CAD build for the part. Positions are in the model's coordinates, mm. Face numbers are marked on the shaded views. Coordinates: 2 decimals unless noted, no trailing zeros. Loops run counter-clockwise (first coordinate to the right, second up) from the corner with the lowest first, then second, coordinate; pieces in that order, holes last. Notation, with made-up numbers: (25, -22) - (52, -22) arc R30 cw to (52, 8) - close; hole circle Ø1 at (49, -11.75). An arc over 180 degrees is marked (long way). Put each result on its own line as item: value.
```python
from build123d import *

# Parameters (mm, degrees)
F0_R     = 12
F1_DEPTH = 6
F2_R     = 18
F3_DEPTH = 2
F5_D     = 1.5
F6_R     = 4
F7_DEPTH = 8.001
F9_D     = 2.5
F9_DEPTH = 18.001


with BuildPart() as f1:
    # F0 (on Top) → F1 (new body)
    with BuildSketch(Plane.XY):
        Circle(F0_R)
    extrude(amount=F1_DEPTH)

    # F2 (on face) → F3 (join)
    with BuildSketch(Plane.XY.offset(6)):
        Circle(F2_R)
    extrude(amount=F3_DEPTH)

    # F5 (through all)
    with Locations(Plane.XY.offset(8)):
        with Locations((-17, 0), (-16.4659137392, 4.2277280818), (-14.8972135607, 8.1898124597), (-12.3924666662, 11.6373008008), (-9.1090555146, 14.3535747335), (-5.2532889044, 16.167960777), (-1.067438832, 16.9664543833), (3.185482348, 16.6988832624), (7.2382479566, 15.3820598919), (10.8362078257, 13.0987251272), (13.7532889044, 9.992349289), (15.8062002601, 6.2581173956), (-16.4659137392, -4.2277280818), (-14.8972135607, -8.1898124597), (-12.3924666662, -11.6373008008), (-9.1090555146, -14.3535747335), (-5.2532889044, -16.167960777), (-1.067438832, -16.9664543833), (3.185482348, -16.6988832624), (7.2382479566, -15.3820598919), (10.8362078257, -13.0987251272), (13.7532889044, -9.992349289), (15.8062002601, -6.2581173956), (16.8659499223, -2.1306649706), (16.8659499223, 2.1306649706)):
            Hole(F5_D / 2)

    # F6 (on face) → F7 (cut, through all)
    with BuildSketch(Plane(origin=(0, 0, 0), x_dir=(1, 0, 0), z_dir=(0, 0, -1))):
        Circle(F6_R)
    extrude(amount=-F7_DEPTH, mode=Mode.SUBTRACT)

    # F9 (through all, one way)
    with BuildSketch(Plane.XZ):
        with Locations((0, 3)):
            Circle(F9_D / 2)
    extrude(amount=-F9_DEPTH, mode=Mode.SUBTRACT)


solid = f1.part
```
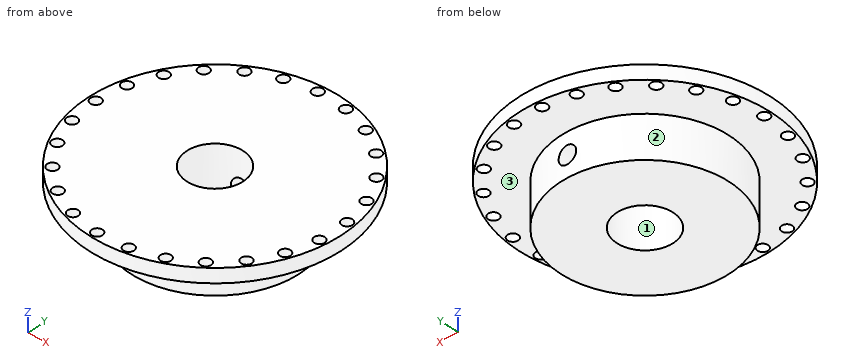
Q1. Pin check, flat tips, straight feed: pin 1 Ø1.7 at (x, y) = (-1.07, -16.97) entering from -Z; pin 2 Ø1.5 at (x, z) = (2.5, 6.5) entering from -Y; pin 3 Ø1.5 at (y, z) = (-7, 4.5) entering from +X. Stop position of each tip, or through.
Determined:
pin 1: z = 6
pin 2: y = -17.91
pin 3: x = 10.24
Q2. Slice it at C-C, the plane z = 5. Give the cut face in (x, y).
Determined:
outline: circle Ø24 at (0, 0); hole circle Ø8 at (0, 0)
Q3. Wall check: L1, parallel to X at y = 16.5, z = 6.75; L2, parallel to Y at x = 3.5, z = 4.5; L3, parallel to Z at x = -16, y = -1. Give the ranges that are in metal, low to high. Write a range as from..to.
Determined:
L1: -7.19..-5.93, -4.58..-1.65, -0.48..2.46, 3.91..7.19
L2: -11.48..-1.94, 1.94..11.48
L3: 6..8
Q4. Mould opens along Y. For the marked faces 1, 2 and 3 say: +Y half, -Y half, draft (parallel to the pull), parting line (faces both ways), or undercut.
Determined:
face 1: undercut
face 2: parting line
face 3: draft
Q5. Slice it at A-A, the plane y = 0. Give the cut face in (x, z), then the cut area to 3 significant figures.
Determined:
outline: (-18, 6) - (-17.75, 6) - (-17.75, 8) - (-18, 8) - close; (-16.25, 6) - (-12, 6) - (-12, 0) - (-4, 0) - (-4, 8) - (-16.25, 8) - close; (4, 0) - (12, 0) - (12, 6) - (18, 6) - (18, 8) - (4, 8) - close
area: 149 mm2
Q6. Slice it at D-D, the plane x = -7. Give the cut face in (y, z).
Determined:
outline: (-16.58, 6) - (-9.75, 6) - (-9.75, 0) - (9.75, 0) - (9.75, 6) - (16.58, 6) - (16.58, 8) - (-16.58, 8) - close
Q7. Slice it at B-B, the plane x = 8.5. Give the cut face in (y, z).
Determined:
outline: (-15.87, 6) - (-8.47, 6) - (-8.47, 0) - (8.47, 0) - (8.47, 6) - (15.87, 6) - (15.87, 8) - (-15.87, 8) - close
